Source: three-view drawing plus pictorial views. Frame: mm from the lowest corner of the part. Give positions to 0.01 mm unless a question says otherwise; leave off trailing zeros. Write each loop counter-clockwise with the first axis right and the second up, starting at its lowest first coordinate (ties: lowest second). Pieces come first, ordered by that corner, then holes.
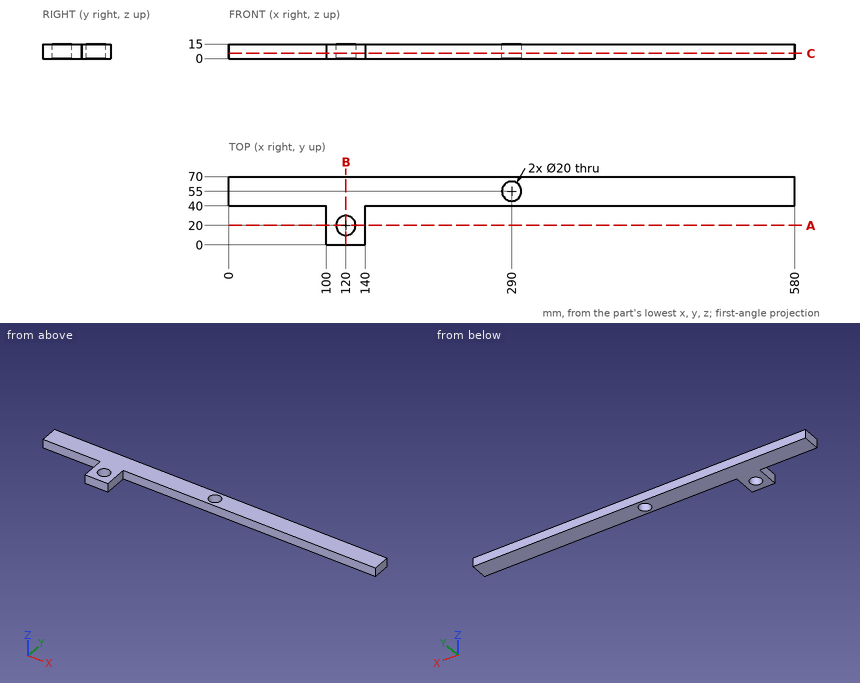
Q1. Section C-C on z = 5.5. Output: boundary loops of the cut face in (x, y), plus the area to 3 significant figures.
Filled sheet:
outline: (0, 40) - (100, 40) - (100, 0) - (140, 0) - (140, 40) - (580, 40) - (580, 70) - (0, 70) - close; hole circle Ø20 at (120, 20); hole circle Ø20 at (290, 55)
area: 18,400 mm2
Q2. Section B-B on x = 120. Output: boundary loops of the cut face in (y, z), plus the area to 3 significant figures.
Filled sheet:
outline: (0, 0) - (10, 0) - (10, 15) - (0, 15) - close; (30, 0) - (70, 0) - (70, 15) - (30, 15) - close
area: 750 mm2
Q3. Section A-A on y = 20. Output: boundary loops of the cut face in (x, z), plus the area to 3 significant figures.
Filled sheet:
outline: (100, 0) - (110, 0) - (110, 15) - (100, 15) - close; (130, 0) - (140, 0) - (140, 15) - (130, 15) - close
area: 300 mm2
Q4. Pin query (flat end, axial travel): P1, Ø1, axis at y = 24, z = 3.5, coming from the -X side; P2, Ø4, axis at y = 18, z = 8.5, coming from the +X side; P3, Ø5, axis at x = 307.5, z = 13, coming from the -Y side; P4, Ø12, axis at x = 290, y = 55, coming from the -Z side (3 decimals). Return the tip coordinate at first contact, or that it passes through.
Filled sheet:
P1: stops at x = 100
P2: stops at x = 140
P3: stops at y = 40
P4: passes through
Q5. Ray query, line 1 along X through (y, z) = (54.5, 4); line 2 along X through (y, z) = (5, 11.75); line 3 along Y through (x, z) = (419, 12). Return the intervals inside material, ascending.
Filled sheet:
line 1: x = 0 to 280.01, 299.99 to 580
line 2: x = 100 to 140
line 3: y = 40 to 70
